Source: three-view drawing plus pictorial views. Frame: mm from the lowest corner of the part. A direction names the side the tool comes from. Coordinates: 2 decimals unless noted, no trailing zeros. Write each loop counter-clockwise with the first axis right and the second up, starting at its lowest first coordinate (ties: lowest second). Pieces come first, ordered by that corner, then holes. Notation, with made-up numbers: (-11.75, 66.25) - (24.25, 66.25) arc R14 ccw to (24.25, 77.25) - close; hole circle Ø3 at (4.5, 7.5). An arc over 180 degrees is marked (long way). Answer as a JSON object with one key per item and string values. Group by question number.
Item 1: Line query: line 1 along X through (y, z) = (6.75, 18) (3 decimals); line 2 along Z through (x, y) = (22, 2); line 3 along Z through (x, y) = (7, 4.75). Output: solid intervals per line, ascending. Write a range as from..to.
Item 2: Set-up query: the marked faces 1, 2, 3 and 4. Return all of +Z, -Z, +X, -X, +Y, -Y with unobstructed straight access to the full face (end or side cutting, diameter ignored); none if empty.
Item 3: Section D-D on y = 2.75. Return loops of the section in (x, z).
Item 4: First-contact query: pin 1 Ø2 at (y, z) = (5.5, 7) entering from -X; pin 2 Ø3 at (x, y) = (22.5, 4) entering from -Z; pin 3 Ø2.5 at (y, z) = (1.5, 13) entering from +X; pin 4 Ø1.8 at (x, z) = (28.5, 18) entering from -Y. Flat tips, straight axial feed; report the tip coordinate or a pass-through.
Item 5: Section C-C on x = 22. Return loops of the section in (y, z), and give its area (3 significant figures).
Item 6: Section A-A on z = 18.75. Return loops of the section in (x, y).
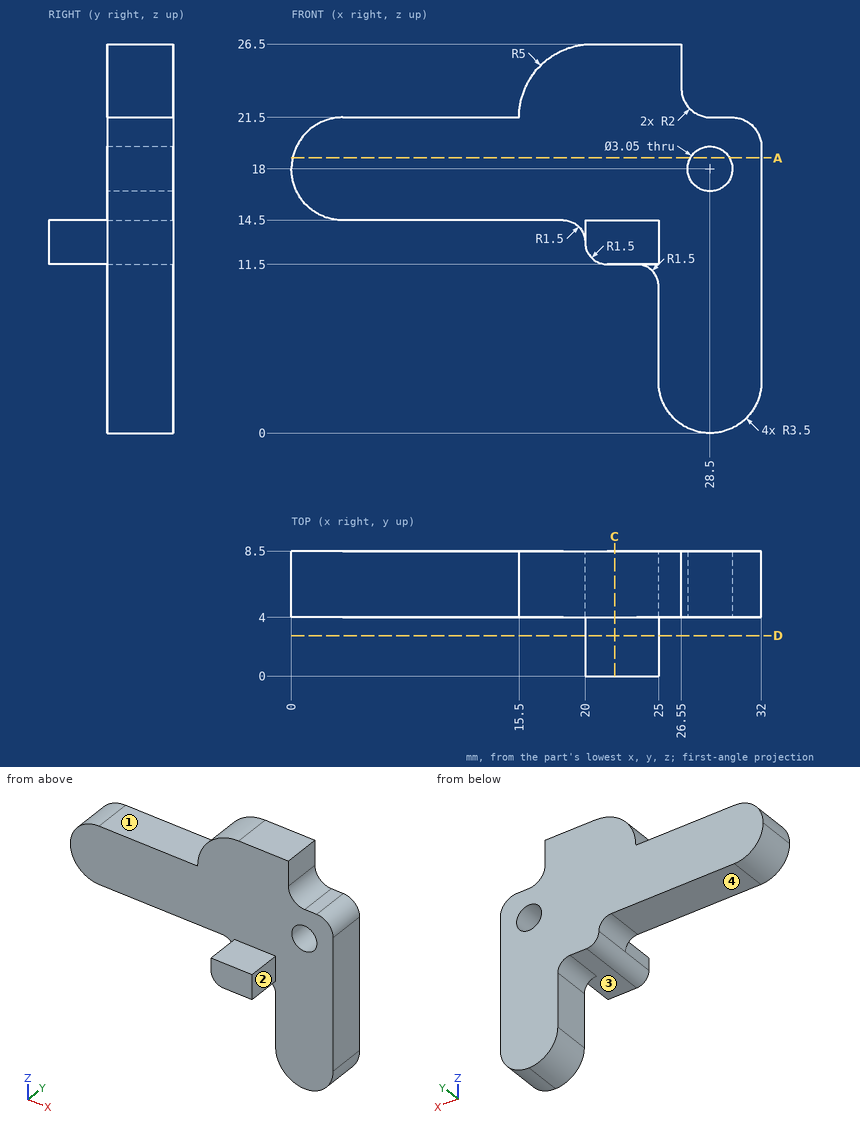
Checks:
{
 "1": {"line 1": "0..26.975, 30.025..32", "line 2": "11.5..14.5", "line 3": "14.5..21.5"},
 "2": {"face 1": "+Z, -X, +Y, -Y", "face 2": "+Z, -Z, +X, -Y", "face 3": "-Z, -X, -Y", "face 4": "-Z, -X, +Y, -Y"},
 "3": {"outline": "(20, 13) arc R1.5 ccw to (21.5, 11.5) - (25, 11.5) - (25, 14.5) - (20, 14.5) - close"},
 "4": {"pin 1": "x = 25", "pin 2": "z = 11.41", "pin 3": "x = 25", "pin 4": "through"},
 "5": {"outline": "(0, 11.5) - (8.5, 11.5) - (8.5, 26.5) - (4, 26.5) - (4, 14.5) - (0, 14.5) - close", "area": "79.5 mm^2"},
 "6": {"outline": "(0.08, 4) - (27.17, 4) - (27.17, 8.5) - (0.08, 8.5) - close; (29.83, 4) - (32, 4) - (32, 8.5) - (29.83, 8.5) - close"}
}
